Geometry: see drawing. Coordinates: mm, zero at the bounding-box minimum. Coordinates: 2 decimals unless noted, no trailing zeros. Order: outer loops, then holes, each group sorted by start corner. A loop starts at its lowest first (then second) coordinate and runs counter-clockwise, first axis right, second up. Notation, with made-up numbers: M 38,78 L 66,78 A22 ccw 66,114 Z; hole C -12,52 d1. An arc over 180 degrees is marked long. Answer in a Markdown table with one row per item.
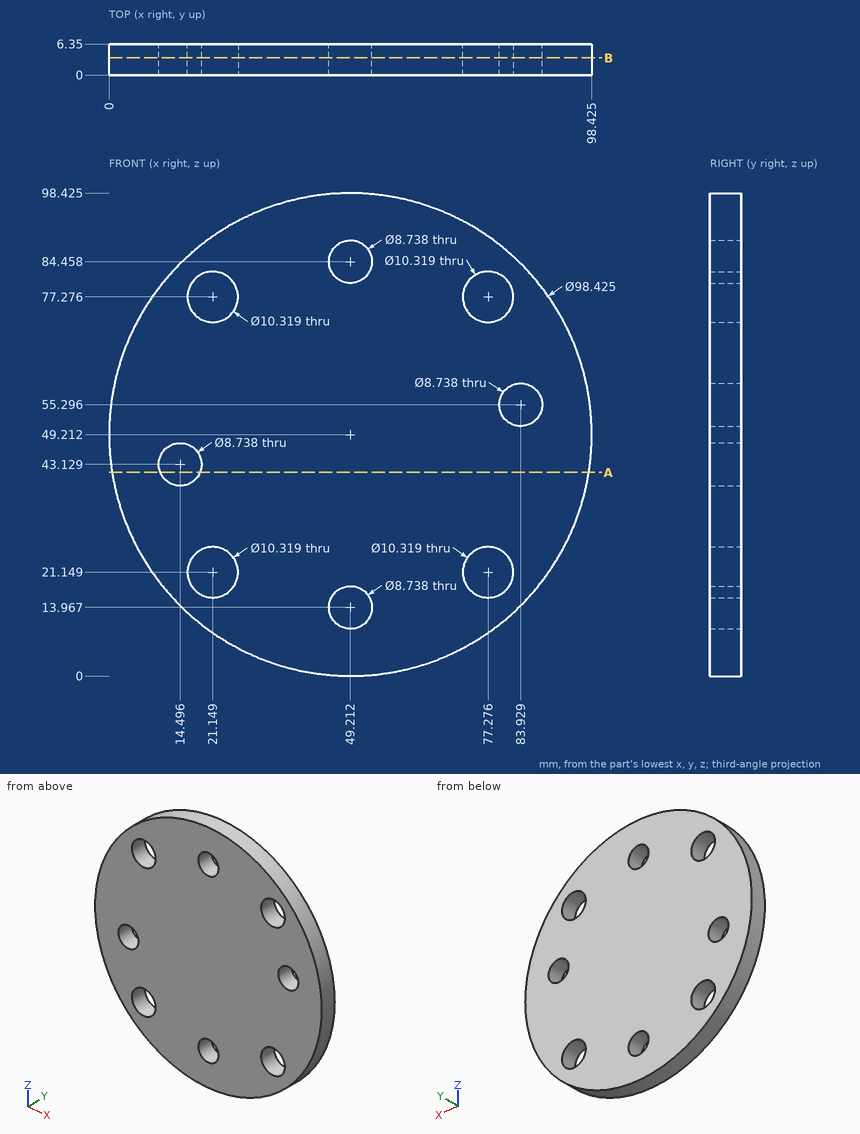
1) Cut plane A-A, the plane z = 41.5. Output: boundary loops of the cut face in (x, y).
Resolved:
| item | result |
|---|---|
| outline | M 0.61,0 L 10.44,0 L 10.44,6.35 L 0.61,6.35 Z; M 18.55,0 L 97.82,0 L 97.82,6.35 L 18.55,6.35 Z |
2) Cut plane B-B, the plane y = 3.5. State how many separate pieces and enclosed holes the cut face has, and give its area (3 significant figures).
Resolved:
| item | result |
|---|---|
| separate pieces | 1 |
| enclosed holes | 8 |
| area | 7,030 mm2 |
3) Contact query for flat-ended pins moving along their axis: pin 1 (1.5 mm diameter, centred on y = 3.5, z = 75, fed in from +X); pin 2 (10 mm diameter, centred on x = 14.5, z = 43.13, fed in from +Y); pin 3 (1.5 mm diameter, centred on y = 2.5, z = 66.5, fed in from +X); pin 4 (1 mm diameter, centred on y = 5.5, z = 87.5, fed in from +X). Output: stop coordinate, or through.
Resolved:
| item | result |
|---|---|
| pin 1 | stops at x = 91.58 |
| pin 2 | stops at y = 6.35 |
| pin 3 | stops at x = 95.56 |
| pin 4 | stops at x = 80.74 |
4) Material intervals for probe 1 along X at (y, z) = (1.5, 25) (1 decimal); probe 2 along Z at (x, y) = (22, 5.5) (1 decimal); probe 3 along X at (y, z) = (1, 21.5) (1 decimal), sorted ascending.
Resolved:
| item | result |
|---|---|
| probe 1 | x = 6.4 to 17.7, 24.6 to 73.8, 80.7 to 92.1 |
| probe 2 | z = 8.2 to 16.1, 26.2 to 72.2, 82.4 to 90.2 |
| probe 3 | x = 8.5 to 16, 26.3 to 72.1, 82.4 to 89.9 |
